Study the drawing (mm; zero at the part's minimum x, y, z) and answer. A direction names the side the tool comes from. Round coordinates to 2 decimals unless told otherwise and drop trailing zeros. Order: outer loops, then holes, each group sorted by start corner. A loop starts at its lowest first (then second) coordinate and runs counter-clockwise, first axis right, second up. Notation, with made-up numbers: (88.5, 59) - (100.5, 59) arc R15 ccw to (100.5, 67) - close; hole circle Ø9 at (14, 44). An arc over 180 degrees is marked (long way). Put each result on its own line as item: value. Start each with the question number.
Q1. Section D-D on y = 66.5 is taken. Give the vertices of the cut face in (x, z) (1 decimal), then the cut area to 3 significant figures.
Q2. Each of these flat-tipped pins is pushed along its axis until it touches: pin 1 Ø3 at (y, z) = (30, 24.69) entering from +X; pin 2 Ø5 at (y, z) = (14, 8.5) entering from -X (1 decimal); pin 3 Ø20.5 at (x, z) = (9, 15.5) entering from +Y. Where does it stop, or does it pass through?
Q3. Find the intervals of material crossed by line 1 along Z through (x, y) = (43.5, 30); line 2 along Y through (x, z) = (37, 10.5); line 3 along Y through (x, z) = (33, 10), in increasing order. Write a range as from..to.
Q4. Which of the six approach directions +Z, -Z, +X, -X, +Y, -Y give full straight-line access (tool end or side, diameter ignored) to the marked faces 1 and 2?
Q5. Section B-B on z = 18 is taken. Give the vertices of the cut face in (x, y) (1 decimal).
Q6. Section A-A on y = 30 is taken. Give the vertices of the cut face in (x, z) (1 decimal).
Q7. Section C-C on x = 4 is taken. Give the vertices of the cut face in (y, z).
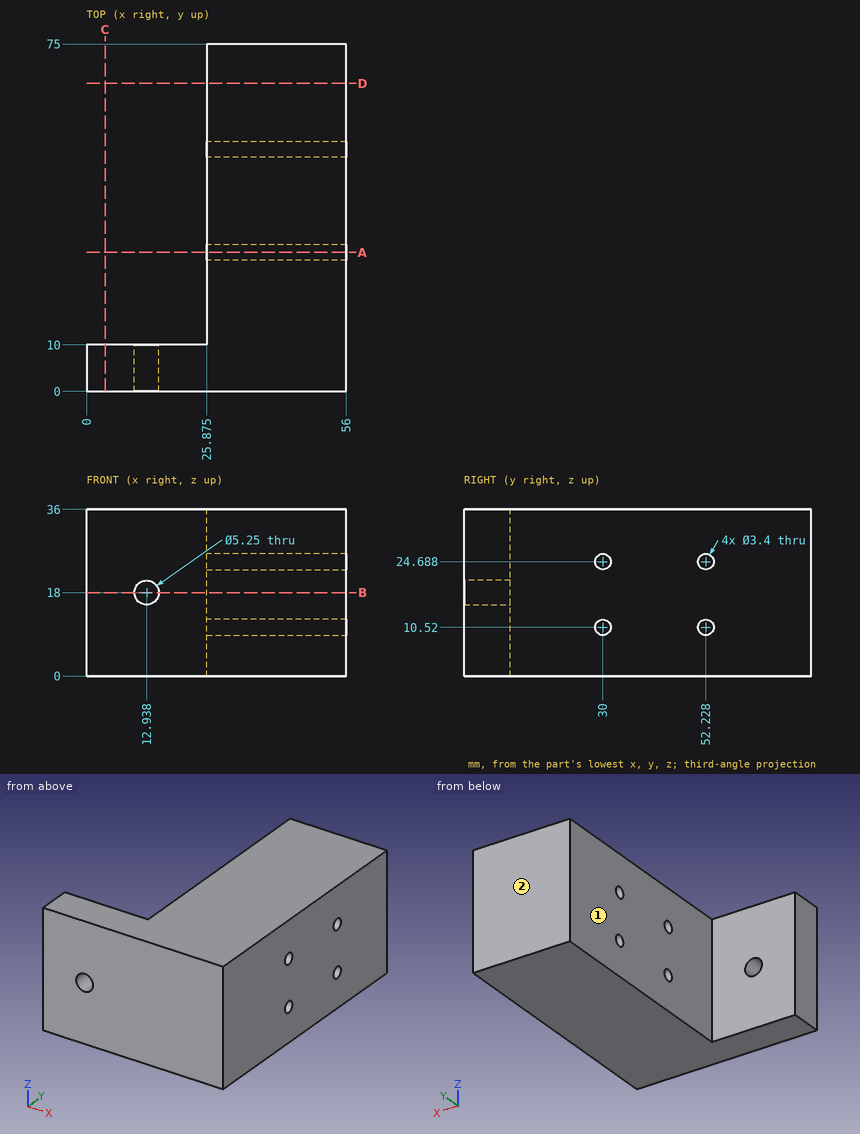
Findings:
1. outline: (25.9, 0) - (56, 0) - (56, 36) - (25.9, 36) - close
1. area: 1,080 mm2
2. pin 1: through
2. pin 2: x = 25.9
2. pin 3: y = 10
3. line 1: 0..8.82, 12.22..22.99, 26.39..36
3. line 2: 0..28.3, 31.7..50.53, 53.93..75
3. line 3: 0..28.38, 31.62..50.61, 53.85..75
4. face 1: +Z, -Z, -X, +Y
4. face 2: +Z, -Z, +X, -X, +Y
5. outline: (0, 0) - (10.3, 0) - (10.3, 10) - (0, 10) - close; (15.6, 0) - (56, 0) - (56, 75) - (25.9, 75) - (25.9, 10) - (15.6, 10) - close
6. outline: (25.9, 0) - (56, 0) - (56, 8.8) - (25.9, 8.8) - close; (25.9, 12.2) - (56, 12.2) - (56, 23) - (25.9, 23) - close; (25.9, 26.4) - (56, 26.4) - (56, 36) - (25.9, 36) - close
7. outline: (0, 0) - (10, 0) - (10, 36) - (0, 36) - close
